from build123d import *

# Parameters (mm, degrees)
CROQUIS1_W                    = 150
CROQUIS1_H                    = 353
SALIENTE_EXTRUIR1_DEPTH       = 4.7625
CROQUIS2_R                    = 3.175
CORTAR_EXTRUIR1_DEPTH         = 192.833082148
CORTAR_EXTRUIR2_REACH         = 193.833
CROQUIS3_R                    = 3
CORTAR_EXTRUIR3_REACH         = 193.833
CROQUIS4_R                    = 5
CORTAR_EXTRUIR7_REACH         = 193.833
TALADRO_ROSCADO_1_2_134_D     = 10.71626
TALADRO_ROSCADO_1_2_134_DEPTH = 35.17
TALADRO_ROSCADO_1_2_134_TIP   = 3.219489309


with BuildPart() as part:
    # Croquis1 → Saliente-Extruir1 (new body)
    with BuildSketch(Plane.XY):
        Rectangle(CROQUIS1_W, CROQUIS1_H)
    extrude(amount=SALIENTE_EXTRUIR1_DEPTH)

    # Croquis2 → Cortar-Extruir1 (cut, through all)
    with BuildSketch(Plane.XY.offset(4.7625)):
        with Locations((-67.5, 170)):
            Circle(CROQUIS2_R)
        with Locations((-32.5, 170)):
            Circle(CROQUIS2_R)
        with Locations((-67.5, 135)):
            Circle(CROQUIS2_R)
        with Locations((-32.5, 135)):
            Circle(CROQUIS2_R)
        with Locations((32.5, 170)):
            Circle(CROQUIS2_R)
        with Locations((67.5, 170)):
            Circle(CROQUIS2_R)
        with Locations((32.5, 135)):
            Circle(CROQUIS2_R)
        with Locations((67.5, 135)):
            Circle(CROQUIS2_R)
        with Locations((-67.5, -135)):
            Circle(CROQUIS2_R)
        with Locations((-32.5, -135)):
            Circle(CROQUIS2_R)
        with Locations((-67.5, -170)):
            Circle(CROQUIS2_R)
        with Locations((-32.5, -170)):
            Circle(CROQUIS2_R)
        with Locations((32.5, -170)):
            Circle(CROQUIS2_R)
        with Locations((32.5, -135)):
            Circle(CROQUIS2_R)
        with Locations((67.5, -135)):
            Circle(CROQUIS2_R)
        with Locations((67.5, -170)):
            Circle(CROQUIS2_R)
    extrude(amount=-CORTAR_EXTRUIR1_DEPTH, mode=Mode.SUBTRACT)

    # Croquis3 → Cortar-Extruir2 (cut, up to next)
    with BuildSketch(Plane(origin=(0, 0, 0), x_dir=(-1, 0, 0), z_dir=(0, 0, -1)), mode=Mode.PRIVATE) as cortar_extruir2_sk1:
        with Locations((-12, 20)):
            Circle(CROQUIS3_R)
    cortar_extruir2_tool1 = extrude(cortar_extruir2_sk1.sketch, amount=-CORTAR_EXTRUIR2_REACH, mode=Mode.PRIVATE) & part.part
    # Croquis3 → Cortar-Extruir2 (cut, up to next)
    with BuildSketch(Plane(origin=(0, 0, 0), x_dir=(-1, 0, 0), z_dir=(0, 0, -1)), mode=Mode.PRIVATE) as cortar_extruir2_sk2:
        with Locations((12, 20)):
            Circle(CROQUIS3_R)
    cortar_extruir2_tool2 = extrude(cortar_extruir2_sk2.sketch, amount=-CORTAR_EXTRUIR2_REACH, mode=Mode.PRIVATE) & part.part
    # Croquis3 → Cortar-Extruir2 (cut, up to next)
    with BuildSketch(Plane(origin=(0, 0, 0), x_dir=(-1, 0, 0), z_dir=(0, 0, -1)), mode=Mode.PRIVATE) as cortar_extruir2_sk3:
        with Locations((12, -20)):
            Circle(CROQUIS3_R)
    cortar_extruir2_tool3 = extrude(cortar_extruir2_sk3.sketch, amount=-CORTAR_EXTRUIR2_REACH, mode=Mode.PRIVATE) & part.part
    # Croquis3 → Cortar-Extruir2 (cut, up to next)
    with BuildSketch(Plane(origin=(0, 0, 0), x_dir=(-1, 0, 0), z_dir=(0, 0, -1)), mode=Mode.PRIVATE) as cortar_extruir2_sk4:
        with Locations((-12, -20)):
            Circle(CROQUIS3_R)
    cortar_extruir2_tool4 = extrude(cortar_extruir2_sk4.sketch, amount=-CORTAR_EXTRUIR2_REACH, mode=Mode.PRIVATE) & part.part
    add(cortar_extruir2_tool1.solids().sort_by_distance((12, 20, 0))[0], mode=Mode.SUBTRACT)
    add(cortar_extruir2_tool2.solids().sort_by_distance((-12, 20, 0))[0], mode=Mode.SUBTRACT)
    add(cortar_extruir2_tool3.solids().sort_by_distance((-12, -20, 0))[0], mode=Mode.SUBTRACT)
    add(cortar_extruir2_tool4.solids().sort_by_distance((12, -20, 0))[0], mode=Mode.SUBTRACT)

    # Croquis4 → Cortar-Extruir3 (cut, up to next)
    with BuildSketch(Plane.XY.offset(4.7625), mode=Mode.PRIVATE) as cortar_extruir3_sk1:
        with Locations((-48.59, -94.11)):
            Circle(CROQUIS4_R)
    cortar_extruir3_tool1 = extrude(cortar_extruir3_sk1.sketch, amount=-CORTAR_EXTRUIR3_REACH, mode=Mode.PRIVATE) & part.part
    add(cortar_extruir3_tool1.solids().sort_by_distance((-48.59, -94.11, 4.7625))[0], mode=Mode.SUBTRACT)

    # Croquis8 → Cortar-Extruir7 (cut, up to next)
    with BuildSketch(Plane.XY.offset(4.7625), mode=Mode.PRIVATE) as cortar_extruir7_sk1:
        with BuildLine():
            Line((75, 114.73), (65, 114.73))
            ThreePointArc((65, 114.73), (37.5, 87.23), (65, 59.73))
            Line((65, 59.73), (75, 59.73))
            Line((75, 59.73), (75, 114.73))
        make_face()
    cortar_extruir7_tool1 = extrude(cortar_extruir7_sk1.sketch, amount=-CORTAR_EXTRUIR7_REACH, mode=Mode.PRIVATE) & part.part
    # Croquis8 → Cortar-Extruir7 (cut, up to next)
    with BuildSketch(Plane.XY.offset(4.7625), mode=Mode.PRIVATE) as cortar_extruir7_sk2:
        with BuildLine():
            Line((75, -53.27), (65, -53.27))
            ThreePointArc((65, -53.27), (37.5, -80.77), (65, -108.27))
            Line((65, -108.27), (75, -108.27))
            Line((75, -108.27), (75, -53.27))
        make_face()
    cortar_extruir7_tool2 = extrude(cortar_extruir7_sk2.sketch, amount=-CORTAR_EXTRUIR7_REACH, mode=Mode.PRIVATE) & part.part
    add(cortar_extruir7_tool1.solids().sort_by_distance((58.604644, 87.23, 4.7625))[0], mode=Mode.SUBTRACT)
    add(cortar_extruir7_tool2.solids().sort_by_distance((58.604644, -80.77, 4.7625))[0], mode=Mode.SUBTRACT)

    # Taladro roscado 1/2-134
    with Locations(Plane.XY.offset(4.7625)):
        with Locations((-48.59, -94.11)):
            Hole(TALADRO_ROSCADO_1_2_134_D / 2, depth=TALADRO_ROSCADO_1_2_134_DEPTH)
            with Locations((0, 0, -(TALADRO_ROSCADO_1_2_134_DEPTH + TALADRO_ROSCADO_1_2_134_TIP / 2))):  # 118° drill point
                Cone(0, TALADRO_ROSCADO_1_2_134_D / 2, TALADRO_ROSCADO_1_2_134_TIP, mode=Mode.SUBTRACT)


solid = part.part
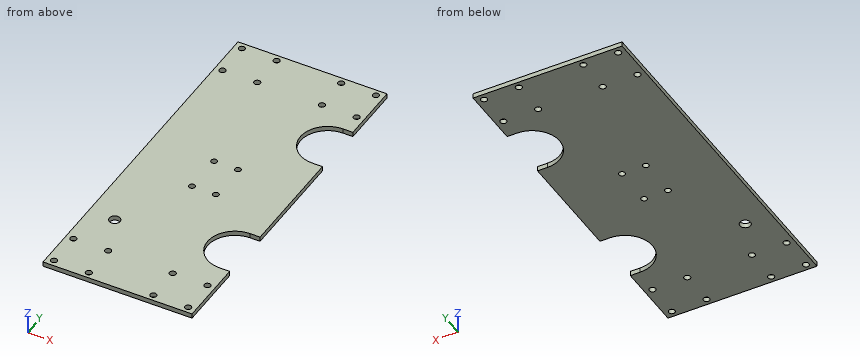
Work out the finished part from the listing and answer in its coordinate system (mm). Coordinates: 2 decimals unless noted, no trailing zeros. Loops run counter-clockwise (first coordinate to the right, second up) from the corner with the lowest first, then second, coordinate; pieces in that order, holes last. Notation, with made-up numbers: (74, 26) -> (129, 26) arc R17 cw to (129, 38) -> close; hole circle Ø1 at (60.25, -35). An arc over 180 degrees is marked (long way). Write each question's results on one line, items separated by ' | '. Start each with the question number.
1) Find section D-D on y = -135. Determine the outline of the cut face in (x, z) (1 decimal), then the cut area to 3 significant figures.
2) A flat-ended cylindrical pin translates along its axis: P1, Ø7.5, axis at x = -67.5, y = -135, coming from the +Z side. Find the tip coordinate at first contact, or state that the pin passes through.
3) Find section B-B on x = -32.5. Determine the outline of the cut face in (y, z) (1 decimal), then the cut area to 3 significant figures.
4) Consider line 1 along X through (y, z) = (-170, 2.7) (3 decimals); line 2 along Y through (x, z) = (12, 3.55); line 3 along Y through (x, z) = (32.5, 1.95) (3 decimals). Determine where each line is inside the solid, lowest interval first.
5) Find section C-C on z = 3.7. Count the separate pieces of the cut face and the enclosed holes in it, then the cut area to 3 significant figures.
6) Find section A-A on x = -48.59. Determine the outline of the cut face in (y, z), then the cut area to 3 significant figures.
Response values:
1) outline: (-75, 0) -> (-70.7, 0) -> (-70.7, 4.8) -> (-75, 4.8) -> close; (-64.3, 0) -> (-35.7, 0) -> (-35.7, 4.8) -> (-64.3, 4.8) -> close; (-29.3, 0) -> (29.3, 0) -> (29.3, 4.8) -> (-29.3, 4.8) -> close; (35.7, 0) -> (64.3, 0) -> (64.3, 4.8) -> (35.7, 4.8) -> close; (70.7, 0) -> (75, 0) -> (75, 4.8) -> (70.7, 4.8) -> close | area: 593 mm^2
2) P1: stops at z = 4.76
3) outline: (-176.5, 0) -> (-173.2, 0) -> (-173.2, 4.8) -> (-176.5, 4.8) -> close; (-166.8, 0) -> (-138.2, 0) -> (-138.2, 4.8) -> (-166.8, 4.8) -> close; (-131.8, 0) -> (131.8, 0) -> (131.8, 4.8) -> (-131.8, 4.8) -> close; (138.2, 0) -> (166.8, 0) -> (166.8, 4.8) -> (138.2, 4.8) -> close; (173.2, 0) -> (176.5, 0) -> (176.5, 4.8) -> (173.2, 4.8) -> close | area: 1,560 mm^2
4) line 1: x = -75 to -70.675, -64.325 to -35.675, -29.325 to 29.325, 35.675 to 64.325, 70.675 to 75 | line 2: y = -176.5 to -23, -17 to 17, 23 to 176.5 | line 3: y = -176.5 to -173.175, -166.825 to -138.175, -131.825 to 131.825, 138.175 to 166.825, 173.175 to 176.5
5) separate pieces: 1 | enclosed holes: 21 | area: 48,800 mm^2
6) outline: (-176.5, 0) -> (-99.47, 0) -> (-99.47, 4.76) -> (-176.5, 4.76) -> close; (-88.75, 0) -> (176.5, 0) -> (176.5, 4.76) -> (-88.75, 4.76) -> close | area: 1,630 mm^2
